The listing builds one solid part. Answer for the finished solid, in the listing's coordinates (mm). A direction names the side the tool comes from. Round coordinates to 2 decimals unless told otherwise and drop trailing zeros. Write each loop counter-clockwise with the first axis right and the second up, starting at its lowest first coordinate (ties: lowest second). Pieces come first, ordered by that corner, then holes. Notation, with made-up numbers: (-1, 32.25) - (18, 32.25) arc R17 cw to (18, 51.25) - close; hole circle Ø5 at (82, -1.75). An arc over 180 degrees is marked (long way). Answer in a Markdown table with one row per item.
from build123d import *

# Parameters (mm, degrees)
F0_R      = 63.5
F1_DEPTH  = 127
F2_R      = 50.8
F3_DEPTH  = 101.6
F4_R      = 38.1
F6_R      = 7.62
F7_DEPTH  = 152.4
F8_R      = 7.62
F9_DEPTH  = 381
F10_R     = 38.1
F11_DEPTH = 381
F12_R     = 13.215582
F13_DEPTH = 25.4


with BuildPart() as f1:
    # F0 (on Right) → F1 (new body)
    with BuildSketch(Plane.YZ):
        Circle(F0_R)
    extrude(amount=F1_DEPTH)

    # F2 (on face) → F3 (cut)
    with BuildSketch(Plane.YZ.offset(127)):
        Circle(F2_R)
    extrude(amount=-F3_DEPTH, mode=Mode.SUBTRACT)

    # F4
    f4_edges = [f1.edges().sort_by_distance(p)[0] for p in [
        (0, -63.5, 0),
    ]]
    fillet(f4_edges, radius=F4_R)

    # F6 (on offset) → F7 (cut)
    with BuildSketch(Plane.XZ.offset(76.2)):
        with Locations((60.656205, 4.460988)):
            Circle(F6_R)
    extrude(amount=-F7_DEPTH, mode=Mode.SUBTRACT)

    # F8 (on Top) → F9 (cut)
    with BuildSketch(Plane.XY):
        with Locations((62.16915, 0)):
            Circle(F8_R)
    extrude(amount=-F9_DEPTH, mode=Mode.SUBTRACT)

    # F10 (on Top) → F11 (cut)
    with BuildSketch(Plane.XY):
        with Locations((71.579769, 0)):
            Circle(F10_R)
    extrude(amount=F11_DEPTH, mode=Mode.SUBTRACT)

    # F12 (on face) → F13 (join)
    with BuildSketch(Plane(origin=(0, 0, 0), x_dir=(0, -1, 0), z_dir=(-1, 0, 0))):
        Circle(F12_R)
    extrude(amount=F13_DEPTH)


solid = f1.part
(1) Section C-C (x = -13.5) is taken. Give the vertices of the cut face in (y, z).
Checked values:
| item | result |
|---|---|
| outline | circle Ø26.43 at (0, 0) |
(2) Find the intervals of material crossed by line 1 (Y direction, x = 92, z = 0); line 2 (Y direction, x = 70.5, z = 48); line 3 (Z direction, x = 105, y = -22), in increasing order.
Checked values:
| item | result |
|---|---|
| line 1 | y = -63.5 to -50.8, 50.8 to 63.5 |
| line 2 | y = -41.57 to -38.08, 38.08 to 41.57 |
| line 3 | z = -59.57 to -45.79, 45.79 to 59.57 |
(3) Section A-A (y = 0) is taken. State how many separate pieces and enclosed holes the cut face has, and give its area (3 significant figures).
Checked values:
| item | result |
|---|---|
| separate pieces | 3 |
| enclosed holes | 0 |
| area | 4,690 mm2 |
(4) Flat-ended cylindrical pins translate along their axes: pin 1 (12 mm diameter, centred on x = 68.5, y = 36.5, fed in from -Z); pin 2 (2 mm diameter, centred on y = 1, z = -28, fed in from +X); pin 3 (17.5 mm diameter, centred on x = 60.66, z = 4.46, fed in from +Y); pin 4 (1.5 mm diameter, centred on y = 6.5, z = -13, fed in from -X). Find the tip coordinate at first contact, or state that the pin passes through.
Checked values:
| item | result |
|---|---|
| pin 1 | stops at z = -55.7 |
| pin 2 | stops at x = 25.4 |
| pin 3 | stops at y = 63.5 |
| pin 4 | stops at x = 0 |
(5) For faces 1 (the cylindrical face through (76.91, 23.44, -45.07)), 2 (the flat face through (127, -29, 43)), 3 (the cylindrical face through (-12.52, 10.49, -8.04)), 4 (the cylindrical face through (89.16, -33.8, 48.34)), determine the directions among +Z, -Z, +X, -X, +Y, -Y from which every point of the face is accessible in a straight line to the end or side of a thin tool.
Checked values:
| item | result |
|---|---|
| face 1 | +X |
| face 2 | +Z, -Z, +X, +Y, -Y |
| face 3 | -X |
| face 4 | +Z |
(6) Section D-D (x = 102) is taken. Give the vertices of the cut face in (y, z), and give its area (3 significant figures).
Checked values:
| item | result |
|---|---|
| outline | (-22.94, 45.33) - (-22.94, 59.21) arc R63.5 ccw (long way) to (22.94, 59.21) - (22.94, 45.33) arc R50.8 cw (long way) to start |
| area | 3,960 mm2 |
(7) For a pull along Z with two mould halves and no side action, classify faces 5 (the flat face through (0, 11, -11)), 6 (the flat face through (25.4, -1, 1)), 7 (the cylindrical face through (81.93, -13.77, -61.99)), 8 (the cylindrical face through (53.044, -56.521, 4.796)) as pulls with the +Z half, pulls with the -Z half, needs draft (parallel to the pull), parting line crosses it, or undercut.
Checked values:
| item | result |
|---|---|
| face 5 | needs draft |
| face 6 | undercut |
| face 7 | parting line crosses it |
| face 8 | undercut |
